Source: three-view drawing plus pictorial views. Frame: mm from the lowest corner of the part. A direction names the side the tool comes from. Give positions to 0.01 mm unless a question says otherwise; leave off trailing zeros. Loops run counter-clockwise (first coordinate to the right, second up) from the corner with the lowest first, then second, coordinate; pieces in that order, holes last. Notation, with made-up numbers: (19, 41.5) -> (48, 41.5) arc R34 ccw to (48, 78.5) -> close; hole circle Ø3 at (39, -5). An arc over 180 degrees is marked (long way). Put each result on its own line as item: value.
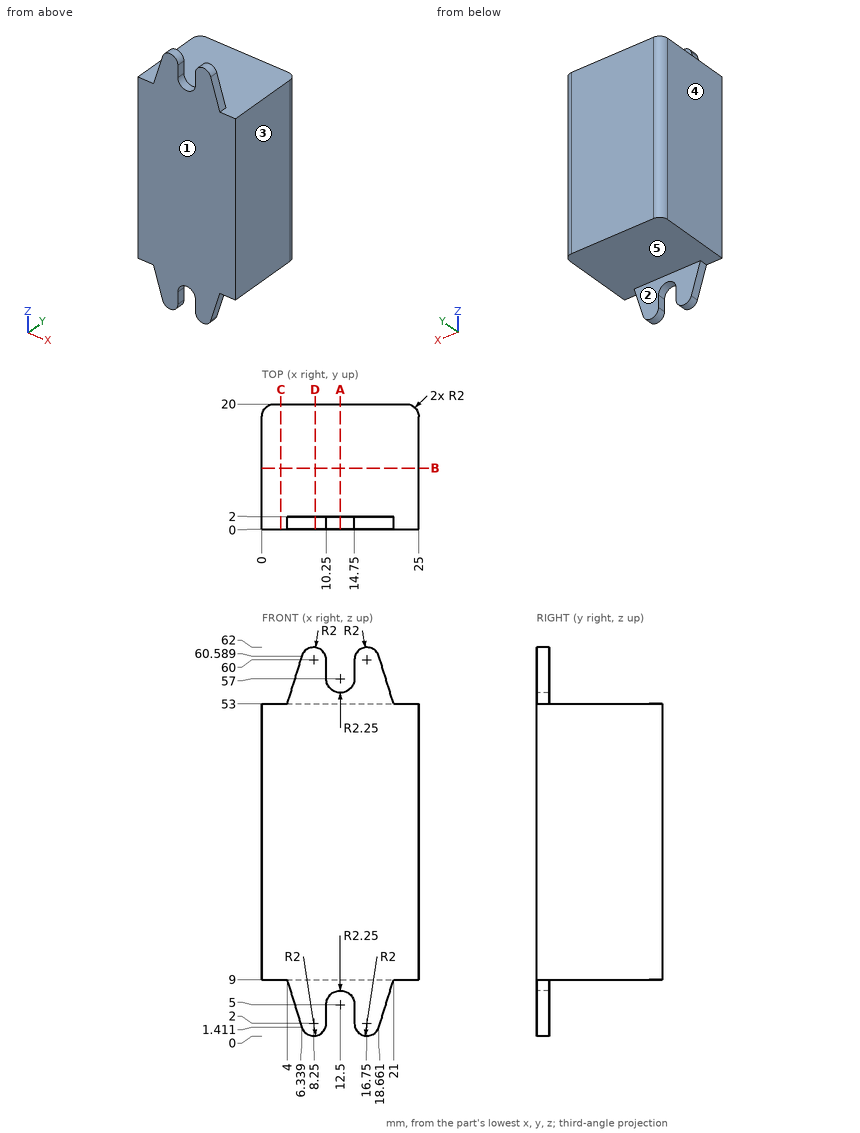
(1) Section B-B on y = 9.75. Return loops of the section in (x, z), then the cut area to 3 significant figures.
Calculated:
outline: (0, 9) -> (25, 9) -> (25, 53) -> (0, 53) -> close
area: 1,100 mm²
(2) Reachability of the marked faces 1 and 2 from +Z, -Z, +X, -X, +Y, -Y: full face, straight path, thin tool, end or side. Return the list, or none.
Calculated:
face 1: +Z, -Z, +X, -X, -Y
face 2: -Z, +X, -X, +Y
(3) Section C-C on x = 3. Return loops of the section in (y, z), then the cut area to 3 significant figures.
Calculated:
outline: (0, 9) -> (20, 9) -> (20, 53) -> (0, 53) -> close
area: 880 mm²
(4) First-contact query: P1, Ø3, axis at y = 17.5, z = 13.5, coming from the -X side; P2, Ø1, axis at y = 1, z = 58.5, coming from the -X side; P3, Ø2, axis at y = 12.5, z = 7, coming from the -X side; P4, Ø2.5, axis at x = 11, z = 57.5, coming from the +Y side. Flat tips, straight axial feed; report the tip coordinate or a pass-through.
Calculated:
P1: stops at x = 0
P2: stops at x = 5.54
P3: passes through
P4: stops at y = 2
(5) Section A-A on x = 12.5. Return loops of the section in (y, z).
Calculated:
outline: (0, 7.25) -> (2, 7.25) -> (2, 9) -> (20, 9) -> (20, 53) -> (2, 53) -> (2, 54.75) -> (0, 54.75) -> close
(6) Section D-D on x = 8.5. Return loops of the section in (y, z).
Calculated:
outline: (0, 0.02) -> (2, 0.02) -> (2, 9) -> (20, 9) -> (20, 53) -> (2, 53) -> (2, 61.98) -> (0, 61.98) -> close
(7) Draft query along X for the marked faces 3, 4 and 5. Return one class per face: released by +X, released by -X, zero draft, split by the parting line, or undercut.
Calculated:
face 3: released by +X
face 4: released by -X
face 5: zero draft
(8) Line query: probe 1 along Z at (x, y) = (5.25, 3.75); probe 2 along Y at (x, z) = (18, 53.5). Output: solid intervals per line, ascending. Write a range as from..to.
Calculated:
probe 1: z = 9..53
probe 2: y = 0..2
